Geometry check sheet. Reference: drawing and pictorial views, mm from the part's lowest x, y, z. Coordinates: 2 decimals unless noted, no trailing zeros. Write each loop counter-clockwise with the first axis right and the second up, starting at its lowest first coordinate (ties: lowest second). Pieces come first, ordered by that corner, then holes. Notation, with made-up numbers: (23.25, -27) -> (57.25, -27) arc R32 ccw to (57.25, 3) -> close; hole circle Ø5 at (-35, 84.25). An arc over 180 degrees is marked (long way). Use a Markdown table: item, result.
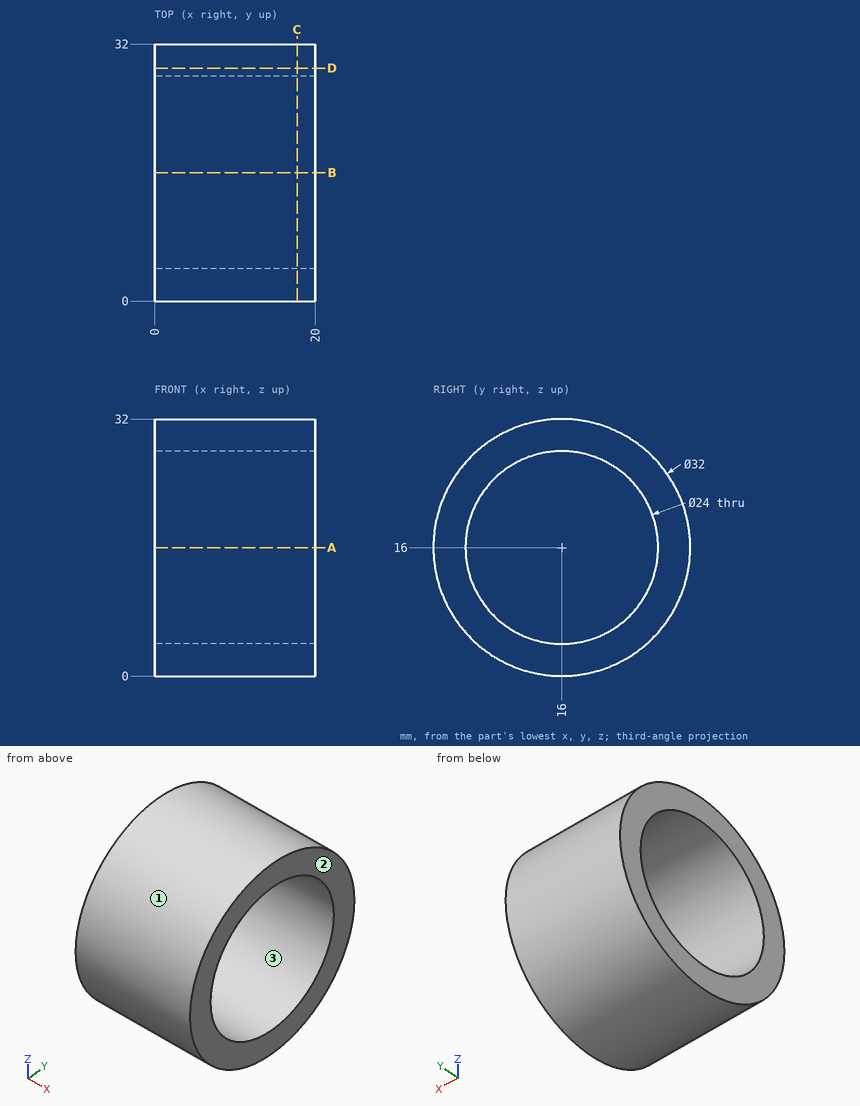
Item 1: Section check C-C on x = 17.75. Record the boundary of the cut face in (y, z), then the cut area to 3 significant figures.
Answer block:
| item | result |
|---|---|
| outline | circle Ø32 at (16, 16); hole circle Ø24 at (16, 16) |
| area | 352 mm^2 |
Item 2: Section check D-D on y = 29. Record the boundary of the cut face in (x, z), then the cut area to 3 significant figures.
Answer block:
| item | result |
|---|---|
| outline | (0, 6.67) -> (20, 6.67) -> (20, 25.33) -> (0, 25.33) -> close |
| area | 373 mm^2 |
Item 3: Mould release check, pull along Z, two halves, no side actions. Record for the marked faces 1, 2 and 3: +Z half, -Z half, draft (parallel to the pull), parting line (faces both ways), or undercut.
Answer block:
| item | result |
|---|---|
| face 1 | parting line |
| face 2 | draft |
| face 3 | undercut |
Item 4: Depth check by flat-ended pin: P1, Ø10, axis at x = 3.5, y = 22.5, coming from the -Z side; P2, Ø2, axis at x = 13.5, z = 18.5, coming from the +Y side; P3, Ø8, axis at x = 2.5, y = 24.5, coming from the -Z side. Enter the tip coordinate at first touch or a pass-through.
Answer block:
| item | result |
|---|---|
| P1 | stops at z = 0.07 |
| P2 | stops at y = 31.93 |
| P3 | stops at z = 0.65 |
Item 5: Section check A-A on z = 16. Record the boundary of the cut face in (x, y), then the cut area to 3 significant figures.
Answer block:
| item | result |
|---|---|
| outline | (0, 0) -> (20, 0) -> (20, 4) -> (0, 4) -> close; (0, 28) -> (20, 28) -> (20, 32) -> (0, 32) -> close |
| area | 160 mm^2 |
Item 6: Thickness scan on L1, parallel to Y at x = 5.5, z = 16; L2, parallel to Y at x = 14.5, z = 26; L3, parallel to Z at x = 15.25, y = 9. Record the ranges inside material, lowest first. Write a range as [from, to].
Answer block:
| item | result |
|---|---|
| L1 | y = [0, 4], [28, 32] |
| L2 | y = [3.51, 9.37], [22.63, 28.49] |
| L3 | z = [1.61, 6.25], [25.75, 30.39] |
